Source: CAD feature listing. Evaluate the final solid. Frame: model axes, mm. Coordinates: 2 decimals unless noted, no trailing zeros. Loops run counter-clockwise (first coordinate to the right, second up) from the corner with the lowest first, then second, coordinate; pieces in that order, holes last.
Item 1: Pin query (flat end, axial travel): pin 1 Ø6 at (x, y) = (50.5, -4) entering from +Z; pin 2 Ø8 at (y, z) = (0, 0) entering from -X (3 decimals); pin 3 Ø4 at (x, z) = (25.5, -3) entering from +Y; pin 4 Ø8 at (x, y) = (48.5, 6) entering from +Z. Return the tip coordinate at first contact, or that it passes through.
Item 2: Section query C-C, the plane x = 69. Return the cut outline in (y, z), then the cut area to 3 significant figures.
Item 3: Pull-direction query (Y, two-part tool) for faces 1 (the cylindrical face through (79.999, -1.017, -7.744)), 2 (the cylindrical face through (82.254, -5.77, -4.424)); classes: +Y half, -Y half, draft (parallel to the pull), parting line (faces both ways), or undercut.
Item 4: Line query: probe 1 along Y at (x, z) = (11.5, -0.25); probe 2 along Z at (x, y) = (50.5, -3); probe 3 along Y at (x, z) = (133, -2.5). Output: solid intervals per line, ascending.
Autodesk Inventor part; units mm, degrees
ref_plane "tube_front_XY" through (0, 0, 0) normal (1, 0, 0) x (0, 0, -1)
ref_plane "tube_front_YZ" through (0, 0, 0) normal (0, 0, -1) x (0, 1, 0)
ref_plane "tube_front_ZX" through (0, 0, 0) normal (0, 1, 0) x (1, 0, 0)
sketch "Sketch_1" plane through (0, 0, 0) normal (0, 0, 1) x (1, 0, 0)
  line L0 (162.2552, 0) -> (0, 0)
  arc A0 (-0.518, 7.0158) -> (-0.518, 6.8362) centre (-0.4282, 6.926) ccw
  line L1 (-0.518, 6.8362) -> (-0.3175, 6.6357)
  line L2 (-0.3175, 6.6357) -> (0, 6.6357)
  line L3 (0, 6.6357) -> (0.635, 7.2708)
  line L4 (0.635, 7.2708) -> (161.6202, 7.2708)
  line L5 (161.6202, 7.2708) -> (162.2552, 6.6357)
  line L6 (162.2552, 6.6357) -> (162.5727, 6.6357)
  line L7 (162.5727, 6.6357) -> (162.7732, 6.8362)
  arc A1 (162.7732, 6.8362) -> (162.7732, 7.0158) centre (162.6834, 6.926) ccw
  line L8 (162.7732, 7.0158) -> (162.1645, 7.6245)
  arc A2 (162.1645, 7.6245) -> (161.7155, 7.8105) centre (161.7154, 7.1755) ccw
  line L9 (161.7155, 7.8105) -> (0.5398, 7.8105)
  arc A3 (0.5398, 7.8105) -> (0.0907, 7.6245) centre (0.5397, 7.1755) ccw
  line L10 (0.0907, 7.6245) -> (-0.518, 7.0158)
revolve "Revolution1" add sketch "Sketch_1" angle 360 about axis through (162.2552, 0, 0) along (1, 0, 0)
ref_plane "tube_front_XY" through (0, 0, 0) normal (1, 0, 0) x (0, 0, -1)
ref_plane "tube_front_YZ" through (0, 0, 0) normal (0, 0, -1) x (0, 1, 0)
ref_plane "tube_front_ZX" through (0, 0, 0) normal (0, 1, 0) x (1, 0, 0)
ref_plane "tube_rear_XY" through (162.2552, 0, 0) normal (1, 0, 0) x (0, 0, -1)
ref_plane "tube_rear_YZ" through (162.2552, 0, 0) normal (0, 0, -1) x (0, 1, 0)
ref_plane "tube_rear_ZX" through (162.2552, 0, 0) normal (0, 1, 0) x (1, 0, 0)
ref_plane "cp1_XY" through (81.1276, 7.8105, 0) normal (1, 0, 0) x (0, 0, -1)
ref_plane "cp1_YZ" through (81.1276, 7.8105, 0) normal (0, 0, -1) x (0, 1, 0)
ref_plane "cp1_ZX" through (81.1276, 7.8105, 0) normal (0, 1, 0) x (1, 0, 0)
ref_plane "cp2_XY" through (81.1276, 0, -7.8105) normal (1, 0, 0) x (0, 0, -1)
ref_plane "cp2_YZ" through (81.1276, 0, -7.8105) normal (0, 0, -1) x (0, 1, 0)
ref_plane "cp2_ZX" through (81.1276, 0, -7.8105) normal (0, 1, 0) x (1, 0, 0)
ref_plane "cp3_XY" through (81.1276, -7.8105, 0) normal (1, 0, 0) x (0, 0, -1)
ref_plane "cp3_YZ" through (81.1276, -7.8105, 0) normal (0, 0, -1) x (0, 1, 0)
ref_plane "cp3_ZX" through (81.1276, -7.8105, 0) normal (0, 1, 0) x (1, 0, 0)
ref_plane "cp4_XY" through (81.1276, 0, 7.8105) normal (1, 0, 0) x (0, 0, -1)
ref_plane "cp4_YZ" through (81.1276, 0, 7.8105) normal (0, 0, -1) x (0, 1, 0)
ref_plane "cp4_ZX" through (81.1276, 0, 7.8105) normal (0, 1, 0) x (1, 0, 0)
properties part number "02-6.3880-nr"
Verdict:
1. pin 1: stops at z = 7.75
1. pin 2: passes through
1. pin 3: stops at y = 7.75
1. pin 4: stops at z = 7.55
2. outline: circle Ø15.62 at (0, 0); hole circle Ø14.54 at (0, 0)
2. area: 25.6 mm2
3. face 1: parting line
3. face 2: undercut
4. probe 1: y = -7.81 to -7.27, 7.27 to 7.81
4. probe 2: z = -7.21 to -6.62, 6.62 to 7.21
4. probe 3: y = -7.4 to -6.83, 6.83 to 7.4
